Autodesk Inventor part; units mm, degrees
ref_plane "YZ Plane" through (0, 0, 0) normal (1, 0, 0) x (0, 1, 0)
ref_plane "XZ Plane" through (0, 0, 0) normal (0, 1, 0) x (-1, 0, 0)
ref_plane "XY Plane" through (0, 0, 0) normal (0, 0, 1) x (1, 0, 0)
sketch "Sketch1" plane through (0, 0, 0) normal (0, 0, 1) x (1, 0, 0)
  line L0 (2.5, 16.45) -> (2.5, -18.55)
  line L1 (2.5, -18.55) -> (0, -18.55)
  line L2 (0, -18.55) -> (0, 18.55)
  line L3 (0, 18.55) -> (4, 18.55)
  line L4 (4, 18.55) -> (4, 16.45)
  line L5 (4, 16.45) -> (2.5, 16.45)
  point P0 (0, 0)
  point P1 (0, 0)
  dimension "d0" = 2.5
  dimension "d1" = 35
  dimension "d2" = 2.1
  dimension "d3" = 4
revolve "Revolution1" add sketch "Sketch1" angle 360 about axis through (0, -18.55, 0) along (0, 1, 0)
fillet "Fillet1" radius 1 1 edges at (-4, 18.55, 0)
sketch "Sketch2" plane through (0, 18.55, 0) normal (0, 1, 0) x (1, 0, 0)
  line L0 (-2.7, 0) -> (-2.7, -0.75)
  line L1 (-2.7, -0.75) -> (-0.75, -0.75)
  line L2 (-0.75, -0.75) -> (-0.75, -2.7)
  line L3 (-0.75, -2.7) -> (0, -2.7)
  line L4 (2.7, -0.75) -> (2.7, 0)
  line L5 (0.75, -2.7) -> (0.75, -0.75)
  line L6 (0, -2.7) -> (0.75, -2.7)
  line L7 (0.75, -0.75) -> (2.7, -0.75)
  line L8 (0.75, 2.7) -> (0, 2.7)
  line L9 (2.7, 0.75) -> (0.75, 0.75)
  line L10 (2.7, 0) -> (2.7, 0.75)
  line L11 (0.75, 0.75) -> (0.75, 2.7)
  line L12 (-2.7, 0.75) -> (-2.7, 0)
  line L13 (-0.75, 2.7) -> (-0.75, 0.75)
  line L14 (0, 2.7) -> (-0.75, 2.7)
  line L15 (-0.75, 0.75) -> (-2.7, 0.75)
  line L16 (-0.75, -2.7) -> (0.75, -2.7)
  line L17 (2.7, -0.75) -> (2.7, 0.75)
  line L18 (-0.75, 2.7) -> (0.75, 2.7)
  line L19 (-2.7, -0.75) -> (-2.7, 0.75)
  point P0 (0, 0)
  dimension "d6" = 0.75
  dimension "d7" = 0.75
  dimension "d8" = 2.7
  dimension "d9" = 2.7
  dimension "d12" = 360
extrude "Extrusion1" cut sketch "Sketch2" against normal blind 1
thread "Thread1"
properties part number "M5x35mm-crosshead"
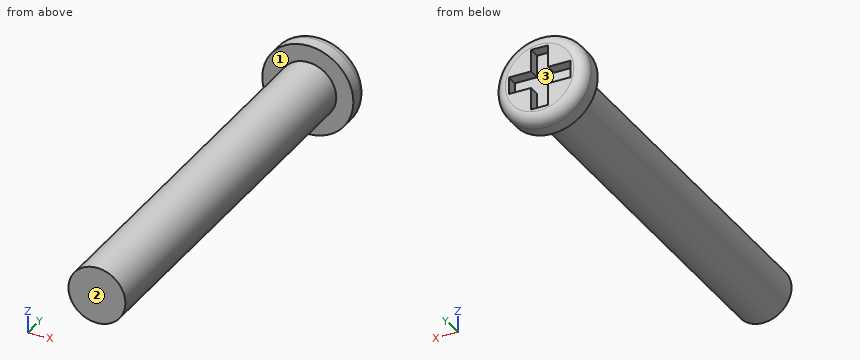
Model file for the job. Use its own axes, mm. Face numbers are marked on the shaded views. A direction names the side the tool comes from. Coordinates: 2 decimals unless noted, no trailing zeros. Loops run counter-clockwise (first coordinate to the right, second up) from the corner with the lowest first, then second, coordinate; pieces in that order, holes last. Notation, with made-up numbers: (-26.75, -22.5) - (-12.75, -22.5) arc R11 cw to (-12.75, -8.5) - close; hole circle Ø2 at (-34.5, 30). An arc over 180 degrees is marked (long way). Answer as a JSON object with one key per item and string values. Group by question number.
(1) Tool access for the marked faces 1, 2 and 3: list every direction of +Z, -Z, +X, -X, +Y, -Y with a clear straight run to the whole face (end or side of a thin tool).
(2) Cut at C-C (y = -15). Give the cut face in (x, z).
(3) Probe line 1 along Y through (x, z) = (2, -2.25); line 2 along Y through (x, z) = (-0.25, -0.25); line 3 along Z through (x, y) = (-0.5, 4). List the from-to ranges inside material, lowest first.
(4) Cut at B-B (x = 0). Give the cut face in (y, z).
(5) Cut at A-A (z = 0). Give the cut face in (x, y), then the cut area to 3 significant figures.
(6) Flat gauge pins, fed straight in: pin 1 (1 mm diameter, centred on x = 0.5, y = -9.5, fed in from -Z); pin 2 (1.5 mm diameter, centred on x = 0.5, z = 0.5, fed in from +Y); pin 3 (0.8 mm diameter, centred on y = 18, z = -1.5, fed in from +X); pin 4 (1 mm diameter, centred on x = -0.5, y = 13.5, fed in from +Z). Where does each tip first touch, or does it go through?
Geometry says:
{
 "1": {"face 1": "-Y", "face 2": "+Z, -Z, +X, -X, -Y", "face 3": "+Y"},
 "2": {"outline": "circle Ø5 at (0, 0)"},
 "3": {"line 1": "y = 16.45 to 18.55", "line 2": "y = -18.55 to 17.55", "line 3": "z = -2.45 to 2.45"},
 "4": {"outline": "(-18.55, -2.5) - (16.45, -2.5) - (16.45, -4) - (17.55, -4) arc R1 ccw to (18.55, -3) - (18.55, -2.7) - (17.55, -2.7) - (17.55, 2.7) - (18.55, 2.7) - (18.55, 3) arc R1 ccw to (17.55, 4) - (16.45, 4) - (16.45, 2.5) - (-18.55, 2.5) - close"},
 "5": {"outline": "(-4, 16.45) - (-2.5, 16.45) - (-2.5, -18.55) - (2.5, -18.55) - (2.5, 16.45) - (4, 16.45) - (4, 17.55) arc R1 ccw to (3, 18.55) - (2.7, 18.55) - (2.7, 17.55) - (-2.7, 17.55) - (-2.7, 18.55) - (-3, 18.55) arc R1 ccw to (-4, 17.55) - close", "area": "186 mm^2"},
 "6": {"pin 1": "stops at z = -2.5", "pin 2": "stops at y = 18.55", "pin 3": "stops at x = 3.8", "pin 4": "stops at z = 2.5"}
}
